Can you work these out from the drawing? Everything is in mm from the part's minimum corner. A direction names the side the tool comes from. Round coordinates to 2 decimals unless told otherwise and drop trailing zeros. Write each loop counter-clockwise with the first axis right and the second up, starting at its lowest first coordinate (ties: lowest second). Pieces come first, ordered by that corner, then holes. Notation, with made-up numbers: (11.5, -39.75) -> (63.5, -39.75) arc R20 cw to (63.5, -2.75) -> close; hole circle Ø9 at (10.25, 88.25). An arc over 180 degrees is marked (long way). Answer as CSV lines item,"result". Start each with the question number.
Q1. Will these pins go through, and if not, where does the flat tip stop? pin 1 Ø3 at (y, z) = (42, 48.5) entering from -X; pin 2 Ø10 at (x, y) = (4.5, 31) entering from +Z; pin 3 Ø5 at (y, z) = (7, 47.5) entering from +X.
Q2. Imagine slicing it at B-B on y = 37. Please give me the cut outline in (x, z).
Q3. Imagine slicing it at A-A on x = 38.1. Please give me the cut outline in (y, z), and give its area (3 significant figures).
Q4. If I drill on line 1 (X direction, y = 38.5, z = 47.5); line 2 (Y direction, x = 58.5, z = 47); line 3 (X direction, y = 44, z = 12.5), over which ranges is the centre line in solid material (lowest first)? Write a range as [from, to].
Q5. Imagine slicing it at C-C on x = 9. Please give me the cut outline in (y, z), and give its area (3 significant figures).
Q6. If we mould it in two halves opening along X, with no side actions, what happens to the marked faces 6, 7 and 8? For each: pulls with the +X half, pulls with the -X half, needs draft (parallel to the pull), parting line crosses it, or undercut.
Q7. For the marked faces 1, 2, 3, 4 and 5, which set-ups out of +Z, -Z, +X, -X, +Y, -Y let a thin tool reach every point of the face, with its end or its side?
Q8. Imagine slicing it at D-D on y = 44. Please give me the cut outline in (x, z).
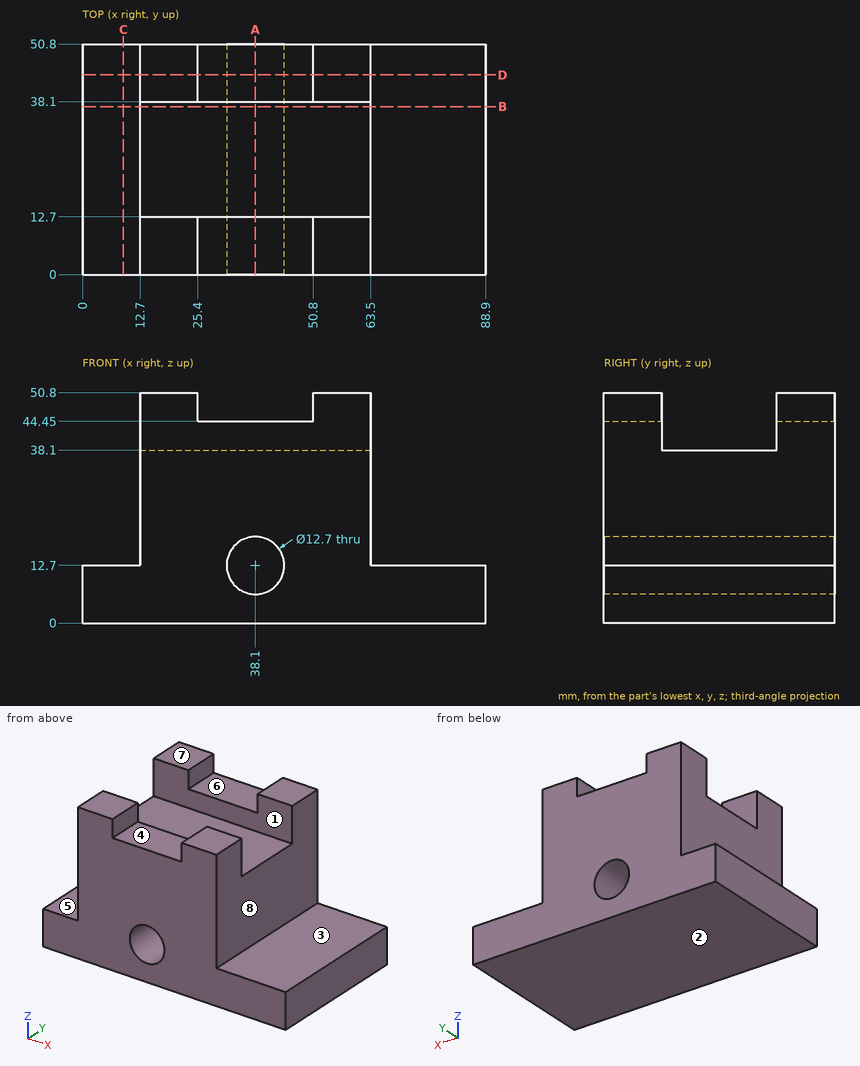
Checks:
1,pin 1,"x = 12.7"
1,pin 2,"z = 12.7"
1,pin 3,"x = 63.5"
2,outline,"(0, 0) -> (88.9, 0) -> (88.9, 12.7) -> (63.5, 12.7) -> (63.5, 38.1) -> (12.7, 38.1) -> (12.7, 12.7) -> (0, 12.7) -> close; hole circle Ø12.7 at (38.1, 12.7)"
3,outline,"(0, 0) -> (50.8, 0) -> (50.8, 6.35) -> (0, 6.35) -> close; (0, 19.05) -> (50.8, 19.05) -> (50.8, 44.45) -> (38.1, 44.45) -> (38.1, 38.1) -> (12.7, 38.1) -> (12.7, 44.45) -> (0, 44.45) -> close"
3,area,"1,450 mm^2"
4,line 1,"[12.7, 25.4], [50.8, 63.5]"
4,line 2,"[0, 12.7], [38.1, 50.8]"
4,line 3,"[0, 31.75], [44.45, 88.9]"
5,outline,"(0, 0) -> (50.8, 0) -> (50.8, 12.7) -> (0, 12.7) -> close"
5,area,"645 mm^2"
6,face 6,"undercut"
6,face 7,"needs draft"
6,face 8,"pulls with the +X half"
7,face 1,"+Z, +X, -X"
7,face 2,"-Z, +X, -X, +Y, -Y"
7,face 3,"+Z, +X, +Y, -Y"
7,face 4,"+Z, +Y, -Y"
7,face 5,"+Z, -X, +Y, -Y"
8,outline,"(0, 0) -> (88.9, 0) -> (88.9, 12.7) -> (63.5, 12.7) -> (63.5, 50.8) -> (50.8, 50.8) -> (50.8, 44.45) -> (25.4, 44.45) -> (25.4, 50.8) -> (12.7, 50.8) -> (12.7, 12.7) -> (0, 12.7) -> close; hole circle Ø12.7 at (38.1, 12.7)"
